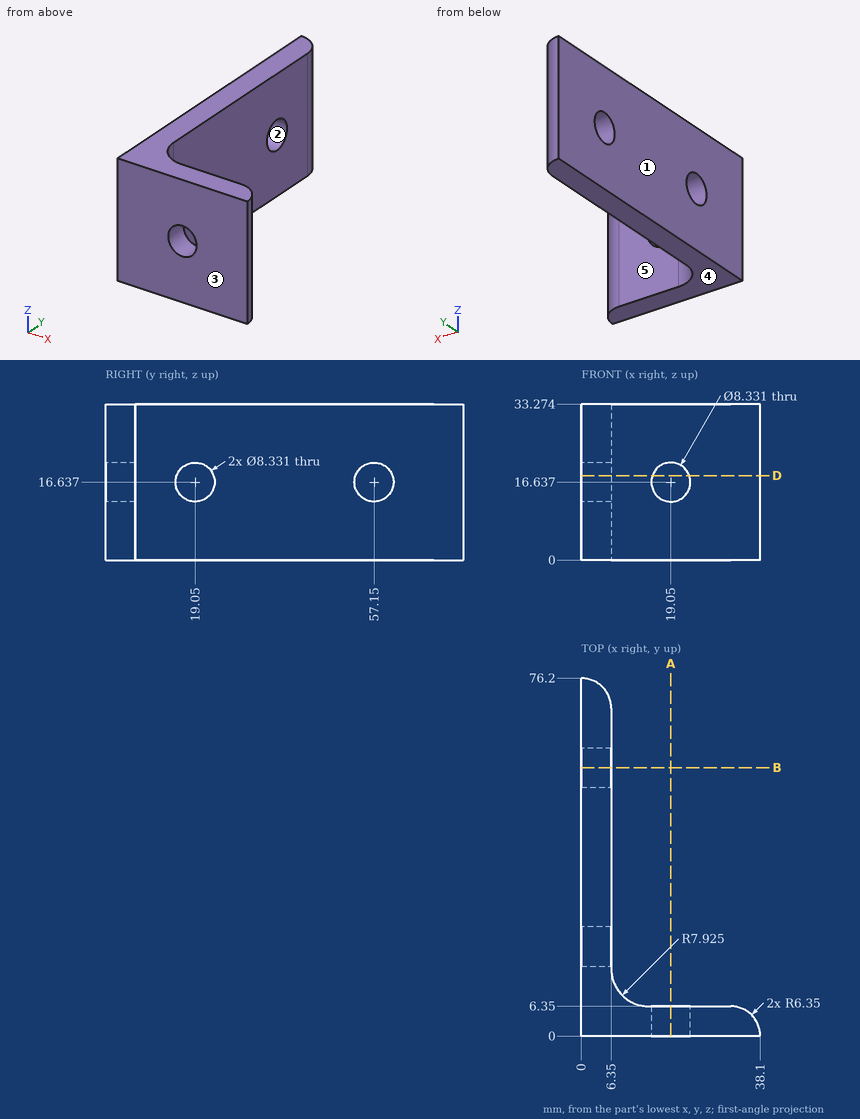
Could you check a few things on this drawing? It's one solid part, dimensions in mm from its lowest x, y, z. A direction names the side the tool comes from. Round coordinates to 2 decimals unless told otherwise and drop trailing zeros. Order: outer loops, then holes, each group sorted by start corner. A loop starts at its lowest first (then second) coordinate and runs counter-clockwise, first axis right, second up.
Q1. Imagine slicing it at D-D, the plane z = 18. State how many separate pieces and enclosed holes the cut face has, then the cut area to 3 significant figures.
Geometry says:
separate pieces: 4
enclosed holes: 0
area: 532 mm2
Q2. Thinking about a two-plate mould opening in Y: for the marked faces 1, 2 and 3, which applies, released by +Y, released by -Y, zero draft, split by the parting line, or undercut?
Geometry says:
face 1: zero draft
face 2: undercut
face 3: released by -Y
Q3. Which directions (+Z, -Z, +X, -X, +Y, -Y) give clear straight access to the entire face, cutting with the end or side of a thin tool? Please do the marked faces 4 and 5.
Geometry says:
face 4: -Z, +X, -X, +Y, -Y
face 5: +Z, -Z, +X, +Y
Q4. Imagine slicing it at A-A, the plane x = 19.05. List the corners of the cut face in (y, z) for me.
Geometry says:
outline: (0, 0) - (6.35, 0) - (6.35, 12.47) - (0, 12.47) - close; (0, 20.8) - (6.35, 20.8) - (6.35, 33.27) - (0, 33.27) - close
Q5. I'm going to push flat-ended pins straight in: P1, Ø12, axis at x = 24, z = 16, coming from the +Y side; P2, Ø1, axis at y = 23, z = 6, coming from the +X side; P3, Ø19, axis at x = 22, z = 20, coming from the +Y side. Where does each tip first touch, or does it pass through?
Geometry says:
P1: stops at y = 6.35
P2: stops at x = 6.35
P3: stops at y = 6.55
Q6. Please list where these lines run through material, in increasing order: probe 1 along Z at (x, y) = (1.5, 57.15); probe 2 along Y at (x, z) = (29.5, 2).
Geometry says:
probe 1: z = 0 to 12.47, 20.8 to 33.27
probe 2: y = 0 to 6.35
